from build123d import *

# Parameters (mm, degrees)
PAD_DEPTH       = 98
SKETCH001_R     = 3
SKETCH001_R_2   = 6
POCKET_DEPTH    = 7
SKETCH002_R     = 9
SKETCH002_R_2   = 2.5
POCKET001_DEPTH = 12


with BuildPart() as part:
    # Sketch → Pad (new body)
    with BuildSketch(Plane.XY):
        with BuildLine():
            Line((6.5, 11.500018), (6.5, 54))
            Line((6.5, 54), (0, 54))
            Line((0, 54), (0, 0))
            Line((0, 0), (50.8, 0))
            Line((50.8, 0), (50.8, 8))
            Line((50.8, 8), (10, 8))
            ThreePointArc((6.5, 11.500018), (7.52512, 9.025133), (10, 8))
        make_face()
    extrude(amount=PAD_DEPTH)

    # Sketch001 → Pocket (cut)
    with BuildSketch(Plane(origin=(0, 0, 0), x_dir=(0, -1, 0), z_dir=(-1, 0, 0))):
        with Locations((-47, 88)):
            Circle(SKETCH001_R)
        with Locations((-7, 78)):
            Circle(SKETCH001_R)
        with Locations((-17, 53)):
            Circle(SKETCH001_R_2)
        with BuildLine():
            Line((-44.000031, 28), (-55, 28))
            Line((-55, 28), (-55, 40))
            Line((-55, 40), (-44.000031, 40))
            ThreePointArc((-44.000031, 28), (-38, 34), (-44.000031, 40))
        make_face()
    extrude(amount=-POCKET_DEPTH, mode=Mode.SUBTRACT)

    # Sketch002 → Pocket001 (cut)
    with BuildSketch(Plane.XZ):
        with Locations((28, 26.5)):
            Circle(SKETCH002_R)
        with Locations((14.564971, 39.935029)):
            Circle(SKETCH002_R_2)
        with Locations((28, 45.5)):
            Circle(SKETCH002_R_2)
        with Locations((41.435029, 39.935029)):
            Circle(SKETCH002_R_2)
        with Locations((14.564971, 13.064971)):
            Circle(SKETCH002_R_2)
        with Locations((28, 7.5)):
            Circle(SKETCH002_R_2)
        with Locations((41.435029, 13.064971)):
            Circle(SKETCH002_R_2)
        with BuildLine():
            Line((6.51, 61.999971), (6.51, 98))
            Line((6.51, 98), (50.8, 98))
            Line((50.8, 98), (50.8, 54))
            Line((50.8, 54), (14.509971, 54))
            ThreePointArc((6.51, 61.999971), (8.853146, 56.343146), (14.509971, 54))
        make_face()
    extrude(amount=-POCKET001_DEPTH, mode=Mode.SUBTRACT)


solid = part.part
The model under review builds one solid part; all positions refer to its coordinate system, in mm. A direction names the side the tool comes from. Round coordinates to 2 decimals unless told otherwise and drop trailing zeros. Write each loop counter-clockwise with the first axis right and the second up, starting at its lowest first coordinate (ties: lowest second). Pieces come first, ordered by that corner, then holes. Notation, with made-up numbers: (73.25, 66.5) - (127.25, 66.5) arc R30 ccw to (127.25, 96.5) - close; hole circle Ø11 at (79, -9). An arc over 180 degrees is marked (long way). One line per item, written item: value. Start each with the question number.
1. Consider section D-D on x = 34.5. Write out the cut boundary in (y, z).
2. Clearance check with flat-ended pins moving along their axes: P1, Ø10, axis at x = 19.5, y = 8.5, coming from the +Z side; P2, Ø8, axis at x = 14.56, z = 39.94, coming from the +Y side; P3, Ø7, axis at y = 47, z = 88, coming from the +X side. State where each tip first meets the part, or that it passes through.
3. The part is to be moulded in two halves that separate along Z. For faces 4 (the face through (25, 0, 37)), 5 (the face through (6, 17, 0)), 6 (the face through (3, 38, 34)), 7 (the face through (8.791, 4.291, 56.406)), say which applies: released by +Z, released by -Z, zero draft, split by the parting line, or undercut.
4. Machinability: for faces 1 (the face through (3, 49, 28)), 2 (the face through (33, 4, 54)), 3 (the face through (35, 8, 33)), which of the approach directions +Z, -Z, +X, -X, +Y, -Y give a long, thin tool a straight path to every point of the face, cutting with its end or side? Answer none if there is none.
5. Consider section B-B on x = 28. Write out the cut boundary in (y, z), and give its area (3 significant figures).
6. Consider section A-A on z = 53. Write out the cut boundary in (x, y), and give its area (3 significant figures).
7. Consider section C-C on y = 47. Write out the cut boundary in (x, z).
8. To check wall thickness, follow L1, parallel to Z at x = 28, y = 4.25; L2, parallel to Z at x = 3.5, y = 7; L3, parallel to X at y = 46, z = 77.5. State the ranges of each line that lie inside material, in increasing order. Write a range as from..to.
Checks:
1. outline: (0, 0) - (8, 0) - (8, 20.28) - (0, 20.28) - close; (0, 32.72) - (8, 32.72) - (8, 54) - (0, 54) - close
2. P1: stops at z = 54
2. P2: stops at y = 8
2. P3: stops at x = 6.5
3. face 4: zero draft
3. face 5: released by -Z
3. face 6: undercut
3. face 7: released by +Z
4. face 1: +X, -X, +Y
4. face 2: +Z, +X, +Y, -Y
4. face 3: +Z, -Z, +X, +Y
5. outline: (0, 0) - (8, 0) - (8, 5) - (0, 5) - close; (0, 10) - (8, 10) - (8, 17.5) - (0, 17.5) - close; (0, 35.5) - (8, 35.5) - (8, 43) - (0, 43) - close; (0, 48) - (8, 48) - (8, 54) - (0, 54) - close
5. area: 208 mm^2
6. outline: (0, 0) - (50.8, 0) - (50.8, 8) - (10, 8) arc R3.5 cw to (6.54, 11) - (0, 11) - close; (0, 23) - (6.5, 23) - (6.5, 54) - (0, 54) - close
6. area: 630 mm^2
7. outline: (0, 0) - (6.5, 0) - (6.5, 28) - (0, 28) - close; (0, 40) - (6.5, 40) - (6.5, 85) - (0, 85) - close; (0, 91) - (6.5, 91) - (6.5, 98) - (0, 98) - close
8. L1: z = 0..5, 10..17.5, 35.5..43, 48..54
8. L2: z = 0..75, 81..98
8. L3: x = 0..6.5
